```python
from build123d import *

# Parameters (mm, degrees)
SKETCH083_W             = 14
SKETCH083_H             = 14
PAD016_DEPTH            = 5
SKETCH084_R             = 2.3
PAD017_DEPTH            = 4.4
FILLET001_R             = 1
SKETCH085_W             = 15.24
SKETCH085_H             = 15.24
PAD018_DEPTH            = 5.8
POCKET009_DEPTH         = 15.241
POCKET010_DEPTH         = 15.621
PAD019_DEPTH            = 3.6
FILLET002_R             = 0.1
CHAMFER_SIZE            = 1
SKETCH089_R             = 0.25
PAD020_DEPTH            = 4
BODY004_PLACEMENT_ANGLE = 180


with BuildPart() as part:
    # Sketch083 → Pad016 (new body)
    with BuildSketch(Plane.XY):
        with Locations((7, 7)):
            Rectangle(SKETCH083_W, SKETCH083_H)
    extrude(amount=PAD016_DEPTH)

    # Sketch084 (on Face6 of Pad016) → Pad017 (join)
    with BuildSketch(Plane.XY.offset(5)):
        with Locations((7, 7)):
            Circle(SKETCH084_R)
    extrude(amount=PAD017_DEPTH)

    # Fillet001
    fillet001_edges = [part.edges().sort_by_distance(p)[0] for p in [
        (4.7, 7, 9.4),
    ]]
    fillet(fillet001_edges, radius=FILLET001_R)

    # Sketch085 (on Face9 of Fillet001) → Pad018 (join)
    with BuildSketch(Plane(origin=(0, 0, 0), x_dir=(1, 0, 0), z_dir=(0, 0, -1))):
        with Locations((7, -7)):
            Rectangle(SKETCH085_W, SKETCH085_H)
    extrude(amount=PAD018_DEPTH)

    # Sketch086 (on Face3 of Pad018) → Pocket009 (cut, through all)
    with BuildSketch(Plane.YZ.offset(14.62)):
        Polygon((-0.62, -5.8), (1.4, -5.8), (-0.62, 0), align=None)
        Polygon((12.6, -5.8), (14.62, -5.8), (14.62, 0), align=None)
    extrude(amount=-POCKET009_DEPTH, mode=Mode.SUBTRACT)

    # Sketch087 → Pocket010 (cut, through all)
    with BuildSketch(Plane.XZ.offset(1)):
        Polygon((12.6, -5.8), (14.62, -5.8), (14.62, 0), align=None)
        Polygon((-0.62, -5.8), (1.4, -5.8), (-0.62, 0), align=None)
    extrude(amount=-POCKET010_DEPTH, mode=Mode.SUBTRACT)

    # Sketch088 (on Face10 of Pocket010) → Pad019 (join)
    with BuildSketch(Plane(origin=(0, 0, -5.8), x_dir=(1, 0, 0), z_dir=(0, 0, -1))):
        Polygon((5.100286, -6.651951), (5.100286, -7.651951), (6.600286, -7.651951), (6.600286, -9.151951), (7.600286, -9.151951), (7.600286, -7.651951), (9.100286, -7.651951), (9.100286, -6.651951), (7.600286, -6.651951), (7.600286, -5.151951), (6.600286, -5.151951), (6.600286, -6.651951), align=None)
    extrude(amount=PAD019_DEPTH)

    # Fillet002
    fillet002_edges = [part.edges().sort_by_distance(p)[0] for p in [
        (6.600286, 9.151951, -7.6),
        (7.600286, 9.151951, -7.6),
        (5.100286, 7.651951, -7.6),
        (9.100286, 7.651951, -7.6),
        (9.100286, 6.651951, -7.6),
        (7.600286, 5.151951, -7.6),
        (6.600286, 5.151951, -7.6),
        (5.100286, 6.651951, -7.6),
    ]]
    fillet(fillet002_edges, radius=FILLET002_R)

    # Chamfer
    chamfer_edges = [part.edges().sort_by_distance(p)[0] for p in [
        (12.6, 7, -5.8),
        (7, 12.6, -5.8),
        (1.4, 7, -5.8),
        (7, 1.4, -5.8),
    ]]
    chamfer(chamfer_edges, length=CHAMFER_SIZE)

    # Sketch089 (on Face36 of Chamfer) → Pad020 (join)
    with BuildSketch(Plane.XY.offset(5)):
        with Locations((11.482716, 10)):
            Circle(SKETCH089_R)
        with Locations((3.493098, 12.4)):
            Circle(SKETCH089_R)
    extrude(amount=PAD020_DEPTH)


with BuildPart() as part_1:
    # Body004 placement: moved
    add(part.part.moved(Location((2, 16, 8))).rotate(Axis((2, 16, 8), (1, 0, 0)), BODY004_PLACEMENT_ANGLE))


solid = part_1.part
```
Input: part model. Units: mm. Frame: model coordinates. A direction names the side the tool comes from. Round coordinates to 2 decimals unless told otherwise and drop trailing zeros. Loops run counter-clockwise (first coordinate to the right, second up) from the corner with the lowest first, then second, coordinate; pieces in that order, holes last. Notation, with made-up numbers: (26, 20.25) - (81, 20.25) arc R11 cw to (81, 31.25) - close; hole circle Ø11 at (34.25, 49). An arc over 180 degrees is marked (long way). One line per item, written item: value. Start each with the question number.
(1) Contact query for flat-ended pins moving along their axis: P1, Ø1.5, axis at x = 15, z = 13, coming from the +Y side; P2, Ø5, axis at x = 4.5, z = 9, coming from the -Y side; P3, Ø1.5, axis at x = 10.5, z = 12.5, coming from the +Y side. Output: stop coordinate, or through.
(2) Section D-D, the plane x = 5. Return loops of the section in (y, z).
(3) Section A-A, the plane y = 6. Return loops of the section in (x, z), plus the area to 3 significant figures.
(4) Section C-C, the plane z = 15.25. Return loops of the section in (x, y).
(5) Section B-B, the plane x = 9. Return loops of the section in (y, z).
(6) Ray query, line 1 (Z direction, x = 13.25, y = 4.75); line 2 (Y direction, x = 11.25, z = 6.75); line 3 (Y direction, x = 8, z = 15.25). Return the intervals inside material, ascending. Write a range as [from, to].
(7) Access query for faces 1 (the flat face through (8, 9.348, 16)), 2 (the flat face through (7, 7, 3)), 3 (the flat face through (9.6, 8, 16)), 4 (the flat face through (10, 9.348, 16)). Directions: +Z, -Z, +X, -X, +Y, -Y. A direction counts if a zero-diameter tool reaches every point of the face in a straight line with its end or side. Return the directions, or none.
Results below:
1. P1: y = 15.14
1. P2: y = 1.38
1. P3: y = 15.31
2. outline: (1.38, 8) - (2, 8) - (2, 3) - (16, 3) - (16, 8) - (16.62, 8) - (14.93, 12.86) - (13.6, 13.8) - (4.4, 13.8) - (3.07, 12.86) - close
3. outline: (1.38, 8) - (2, 8) - (2, 3) - (13.23, 3) - (13.23, -1) - (13.73, -1) - (13.73, 3) - (16, 3) - (16, 8) - (16.62, 8) - (14.93, 12.86) - (13.6, 13.8) - (4.4, 13.8) - (3.07, 12.86) - close
3. area: 148 mm^2
4. outline: (7.1, 8.45) arc R0.1 ccw to (7.2, 8.35) - (8.6, 8.35) - (8.6, 6.95) arc R0.1 ccw to (8.7, 6.85) - (9.5, 6.85) arc R0.1 ccw to (9.6, 6.95) - (9.6, 8.35) - (11, 8.35) arc R0.1 ccw to (11.1, 8.45) - (11.1, 9.25) arc R0.1 ccw to (11, 9.35) - (9.6, 9.35) - (9.6, 10.75) arc R0.1 ccw to (9.5, 10.85) - (8.7, 10.85) arc R0.1 ccw to (8.6, 10.75) - (8.6, 9.35) - (7.2, 9.35) arc R0.1 ccw to (7.1, 9.25) - close
5. outline: (1.38, 8) - (2, 8) - (2, 3) - (6.7, 3) - (6.7, -0.4) arc R1 ccw to (7.7, -1.4) - (10.3, -1.4) arc R1 ccw to (11.3, -0.4) - (11.3, 3) - (16, 3) - (16, 8) - (16.62, 8) - (14.93, 12.86) - (13.6, 13.8) - (10.85, 13.8) - (10.85, 17.4) - (6.85, 17.4) - (6.85, 13.8) - (4.4, 13.8) - (3.07, 12.86) - close
6. line 1: [3, 13.8]
6. line 2: [2, 16]
6. line 3: [8.35, 9.35]
7. face 1: +Z, -X, +Y
7. face 2: -Z
7. face 3: +Z, +X, -Y
7. face 4: +Z, +X, +Y
